```python
from build123d import *

# Parameters (mm, degrees)
SKETCH_1_R                  = 3.15
EXTRUDE_1_DEPTH             = 4
SM_EDGE_FLANGE_1_DEPTH      = 50
SM_EDGE_FLANGE_1_BEND_DEPTH = 50
SKETCH_21_R                 = 1.65
CUT_EXTRUDE_1_DEPTH         = 161.903697907
SKETCH_22_R                 = 1.65
CUT_EXTRUDE_2_DEPTH         = 161.903697907


# Sheet-metal steps are written as plain solids
with BuildPart() as part:
    # Sketch 1 → 凸台-拉伸1 (new body)
    with BuildSketch(Plane(origin=(0, 0, 0), x_dir=(1, 0, 0), z_dir=(0, 1, 0))):
        with BuildLine():
            Line((-25, 65), (-45.371050591, 21.011134388))
            ThreePointArc((-45.371050591, 21.011134388), (-35.355339059, -35.355339059), (21.011134388, -45.371050591))
            Line((21.011134388, -45.371050591), (65, -25))
            Line((65, -25), (65, 25))
            Line((65, 25), (37.660706721, 37.660706721))
            Line((37.660706721, 37.660706721), (25, 65))
            Line((25, 65), (-25, 65))
        make_face()
        with Locations(Location((0, 41, 0), (0, 0, 270))):
            Circle(SKETCH_1_R, mode=Mode.SUBTRACT)
        with Locations(Location((0, -41, 0), (0, 0, 270))):
            Circle(SKETCH_1_R, mode=Mode.SUBTRACT)
        with Locations(Location((-41, 0, 0), (0, 0, 270))):
            Circle(SKETCH_1_R, mode=Mode.SUBTRACT)
        with BuildLine():
            ThreePointArc((29, -24), (27.535533906, -27.535533906), (24, -29))
            Line((24, -29), (-24, -29))
            ThreePointArc((-24, -29), (-27.535533906, -27.535533906), (-29, -24))
            Line((-29, -24), (-29, 24))
            ThreePointArc((-29, 24), (-27.535533906, 27.535533906), (-24, 29))
            Line((-24, 29), (24, 29))
            ThreePointArc((24, 29), (27.535533906, 27.535533906), (29, 24))
            Line((29, 24), (29, -24))
        make_face(mode=Mode.SUBTRACT)
        with Locations(Location((41, 0, 0), (0, 0, 270))):
            Circle(SKETCH_1_R, mode=Mode.SUBTRACT)
    extrude(amount=EXTRUDE_1_DEPTH)

    # 边线-法兰1 section (across the edge) → 边线-法兰1 (add)
    with BuildSketch(Plane(origin=(69, 4, 25), x_dir=(-1, 0, 0), z_dir=(0, 0, -1))):
        with BuildLine():
            Line((-4, 4), (-4, 76))
            Line((-4, 76), (0, 76))
            Line((0, 76), (0, 4))
            ThreePointArc((0, 4), (1.171572875, 1.171572875), (4, 0))
            Line((4, 0), (4, -4))
            ThreePointArc((4, -4), (-1.656854249, -1.656854249), (-4, 4))
        make_face()
    extrude(amount=SM_EDGE_FLANGE_1_DEPTH)

    # 边线-法兰1 section 2 (across the edge) → 边线-法兰1 bend (add)
    with BuildSketch(Plane(origin=(25, 4, -69), x_dir=(0, 0, 1), z_dir=(-1, 0, 0))):
        with BuildLine():
            Line((-4, 4), (-4, 76))
            Line((-4, 76), (0, 76))
            Line((0, 76), (0, 4))
            ThreePointArc((0, 4), (1.171572875, 1.171572875), (4, 0))
            Line((4, 0), (4, -4))
            ThreePointArc((4, -4), (-1.656854249, -1.656854249), (-4, 4))
        make_face()
    extrude(amount=SM_EDGE_FLANGE_1_BEND_DEPTH)

    # 草图21 → 切除-拉伸1 (cut, through all)
    with BuildSketch(Plane.XY.offset(-69)):
        with Locations((-12.5, 40.5)):
            Circle(SKETCH_21_R)
        with Locations(Location((12.5, 40.5, 0), (0, 0, 180))):
            Circle(SKETCH_21_R)
        with Locations((12.5, 15.5)):
            Circle(SKETCH_21_R)
        with Locations(Location((-12.5, 15.5, 0), (0, 0, 180))):
            Circle(SKETCH_21_R)
    extrude(amount=-CUT_EXTRUDE_1_DEPTH, mode=Mode.SUBTRACT)

    # 草图22 → 切除-拉伸2 (cut, through all)
    with BuildSketch(Plane.ZY.offset(-69)):
        with Locations(Location((-12.5, 40.5, 0), (0, 0, 270))):
            Circle(SKETCH_22_R)
        with Locations(Location((12.5, 40.5, 0), (0, 0, 90))):
            Circle(SKETCH_22_R)
        with Locations(Location((12.5, 15.5, 0), (0, 0, 270))):
            Circle(SKETCH_22_R)
        with Locations(Location((-12.5, 15.5, 0), (0, 0, 90))):
            Circle(SKETCH_22_R)
    extrude(amount=-CUT_EXTRUDE_2_DEPTH, mode=Mode.SUBTRACT)


solid = part.part
```
CAD build for the part. Positions are in the model's coordinates, mm. A direction names the side the tool comes from. Round coordinates to 2 decimals unless told otherwise and drop trailing zeros. Write each loop counter-clockwise with the first axis right and the second up, starting at its lowest first coordinate (ties: lowest second). Pieces come first, ordered by that corner, then holes. Notation, with made-up numbers: (11.5, 80) - (25.5, 80) arc R21 cw to (25.5, 114) - close; hole circle Ø9 at (-32.5, 65). An arc over 180 degrees is marked (long way). Return JSON: item names as keys, results as strings. Group by question number.
Item 1: 3-axis set-ups, long thin cutter, end or side, ignore diameter. For faces 5 (the face through (32, 4, -8)), 6 (the face through (0, 2, -29)), 7 (the face through (0, 45, -69)): which of +Z, -Z, +X, -X, +Y, -Y reach the whole face in a straight line?
Item 2: Flat gauge pins, fed straight in: pin 1 Ø1.2 at (y, z) = (3, -12) entering from -X; pin 2 Ø2 at (x, y) = (-2, 2) entering from +Z; pin 3 Ø1 at (x, z) = (48, -4.5) entering from +Y; pin 4 Ø2.5 at (x, y) = (67.5, 35.5) entering from +Z. Where does each tip first touch, or does it go through?
Item 3: Mould opens along Z. For faces 1 (the face through (27, 2, -28)), 2 (the face through (0.35, 2.281, -70.594)), 3 (the face through (0.35, 5.203, -67.859)), 4 (the face through (28, 2, 27)) say: +Z half, -Z half, draft (parallel to the pull), parting line (faces both ways), or undercut.
Item 4: Probe probe 1 along Z at (x, y) = (70.15, 40.5); probe 2 along X at (y, z) = (2.55, 0); probe 3 along X at (y, z) = (40, -70). List the from-to ranges inside material, lowest first.
Item 5: Band-saw the part on D-D on x = 0. List the corners of the cut face in (y, z).
Item 6: Band-saw the part on B-B on z = -40. List the corners of the cut face in (x, y), plus the area to 3 significant figures.
Item 7: Band-saw the part on C-C on y = 67.5. List the corners of the cut face in (x, z).
Item 8: Band-saw the part on A-A on y = 15.5. List the corners of the cut face in (x, z), plus the area to 3 significant figures.
Resolved:
{
 "1": {"face 5": "+Z, -X, +Y", "face 6": "+Y, -Y", "face 7": "+Z, +X, -X, +Y"},
 "2": {"pin 1": "stops at x = -48.68", "pin 2": "stops at z = 49.99", "pin 3": "stops at y = 4", "pin 4": "passes through"},
 "3": {"face 1": "undercut", "face 2": "-Z half", "face 3": "+Z half", "face 4": "undercut"},
 "4": {"probe 1": "z = -25 to -14.15, -10.85 to 10.85, 14.15 to 25", "probe 2": "x = -50 to -44.15, -37.85 to -29, 29 to 37.85, 44.15 to 70.86", "probe 3": "x = -25 to -14.07, -10.93 to 10.93, 14.07 to 25"},
 "5": {"outline": "(0, -65) arc R8 ccw to (8, -73) - (80, -73) - (80, -69) - (8, -69) arc R4 cw to (4, -65) - (4, -44.15) - (0, -44.15) - close; (0, -37.85) - (4, -37.85) - (4, -29) - (0, -29) - close; (0, 29) - (4, 29) - (4, 37.85) - (0, 37.85) - close; (0, 44.15) - (4, 44.15) - (4, 50) - (0, 50) - close"},
 "6": {"outline": "(-36.58, 0) - (-2.99, 0) - (-2.99, 4) - (-36.58, 4) - close; (2.99, 0) - (36.58, 0) - (36.58, 4) - (2.99, 4) - close", "area": "269 mm²"},
 "7": {"outline": "(-25, -73) - (25, -73) - (25, -69) - (-25, -69) - close; (69, -25) - (73, -25) - (73, 25) - (69, 25) - close"},
 "8": {"outline": "(-25, -73) - (-14.15, -73) - (-14.15, -69) - (-25, -69) - close; (-10.85, -73) - (10.85, -73) - (10.85, -69) - (-10.85, -69) - close; (14.15, -73) - (25, -73) - (25, -69) - (14.15, -69) - close; (69, -25) - (73, -25) - (73, -14.15) - (69, -14.15) - close; (69, -10.85) - (73, -10.85) - (73, 10.85) - (69, 10.85) - close; (69, 14.15) - (73, 14.15) - (73, 25) - (69, 25) - close", "area": "347 mm²"}
}
